Design review of the part built by this model. Coordinates are the model's own, in mm. Face numbers are marked on the shaded views. A direction names the side the tool comes from. Coordinates: 2 decimals unless noted, no trailing zeros. Write each loop counter-clockwise with the first axis right and the second up, starting at its lowest first coordinate (ties: lowest second). Pieces come first, ordered by that corner, then holes. Notation, with made-up numbers: (37, 63) -> (46, 63) arc R27 cw to (46, 80) -> close; hole circle Ø5 at (-29.75, 11.25). An arc over 180 degrees is marked (long way). Answer in a Markdown table with one row per item. Add a question column.
Item 1: Clearance check with flat-ended pins moving along their axes: P1, Ø4, axis at x = 12.7, z = -12.7, coming from the -Y side; P2, Ø2, axis at x = 5.5, z = -1, coming from the +Y side; P3, Ø1.5, axis at x = 15.5, y = -16, coming from the -Z side; P4, Ø5.5, axis at x = 8, z = -10, coming from the +Y side. State where each tip first meets the part, or that it passes through.
Item 2: Draft analysis for pull direction X (two halves, no side actions). For the marked faces 1, 2, 3 and 4, state which applies: released by +X, released by -X, zero draft, split by the parting line, or undercut.
Item 3: Take a section at A-A, the plane z = -12.7. Write out the cut boundary in (x, y).
Item 4: Take a section at C-C, the plane x = 12.7. Write out the cut boundary in (y, z).
Item 5: Take a section at D-D, the plane y = -22. Write out the cut boundary in (x, z), and give its area (3 significant figures).
Item 6: To check wall thickness, follow line 1 (Y direction, x = 12.7, z = -0.5); line 2 (X direction, y = -22, z = -12.7); line 3 (Z direction, x = 16.75, y = -1.5). State the ranges of each line that lie inside material, in increasing order.
Item 7: Take a section at B-B, the plane y = -12.7. Write out the cut boundary in (x, z), and give its area (3 significant figures).
Item 8: For the marked faces 5 and 6, list the 3-axis set-ups (+Z, -Z, +X, -X, +Y, -Y) from which the entire face can be reached by the end or side of a thin tool; tool diameter is ignored.
from build123d import *

# Parameters (mm, degrees)
SKETCH1_W           = 25.4
SKETCH1_H           = 25.4
SKETCH1_R           = 3.429
BOSS_EXTRUDE1_DEPTH = 2.54
SKETCH3_W           = 25.4
SKETCH3_H           = 5.08
BOSS_EXTRUDE2_DEPTH = 25.4
SKETCH4_R           = 3.429
CUT_EXTRUDE1_DEPTH  = 5.08
FILLET1_R           = 2.54


with BuildPart() as part:
    # Sketch1 → Boss-Extrude1 (new, symmetric)
    with BuildSketch(Plane.XY):
        with Locations((12.7, -12.7)):
            Rectangle(SKETCH1_W, SKETCH1_H)
        with Locations((12.7, -12.7)):
            Circle(SKETCH1_R, mode=Mode.SUBTRACT)
    extrude(amount=BOSS_EXTRUDE1_DEPTH, both=True)

    # Sketch3 → Boss-Extrude2 (add)
    with BuildSketch(Plane.XY.offset(2.54)):
        with Locations((12.7, -22.86)):
            Rectangle(SKETCH3_W, SKETCH3_H)
    extrude(amount=-BOSS_EXTRUDE2_DEPTH)

    # Sketch4 → Cut-Extrude1 (cut)
    with BuildSketch(Plane(origin=(0, -20.32, 0), x_dir=(1, 0, 0), z_dir=(0, 1, 0))):
        with Locations(Location((12.7, 12.7, 0), (0, 0, 270))):
            Circle(SKETCH4_R)
    extrude(amount=-CUT_EXTRUDE1_DEPTH, mode=Mode.SUBTRACT)

    # Fillet1
    fillet1_edges = [part.edges().sort_by_distance(p)[0] for p in [
        (12.7, -20.32, -2.54),
    ]]
    fillet(fillet1_edges, radius=FILLET1_R)


solid = part.part
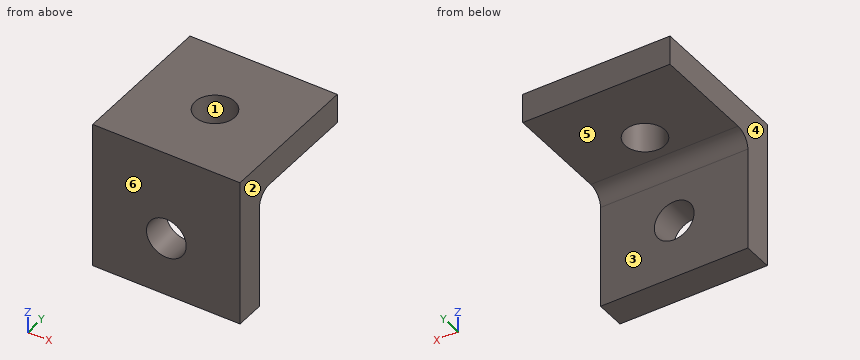
Answers:
| question | item | result |
|---|---|---|
| 1 | P1 | passes through |
| 1 | P2 | stops at y = 0 |
| 1 | P3 | stops at z = -2.54 |
| 1 | P4 | stops at y = -20.32 |
| 2 | face 1 | undercut |
| 2 | face 2 | released by +X |
| 2 | face 3 | zero draft |
| 2 | face 4 | released by -X |
| 3 | outline | (0, -25.4) -> (9.27, -25.4) -> (9.27, -20.32) -> (0, -20.32) -> close; (16.13, -25.4) -> (25.4, -25.4) -> (25.4, -20.32) -> (16.13, -20.32) -> close |
| 4 | outline | (-25.4, -22.86) -> (-20.32, -22.86) -> (-20.32, -16.13) -> (-25.4, -16.13) -> close; (-25.4, -9.27) -> (-20.32, -9.27) -> (-20.32, -5.08) arc R2.54 cw to (-17.78, -2.54) -> (-16.13, -2.54) -> (-16.13, 2.54) -> (-25.4, 2.54) -> close; (-9.27, -2.54) -> (0, -2.54) -> (0, 2.54) -> (-9.27, 2.54) -> close |
| 5 | outline | (0, -22.86) -> (25.4, -22.86) -> (25.4, 2.54) -> (0, 2.54) -> close; hole circle Ø6.86 at (12.7, -12.7) |
| 5 | area | 608 mm^2 |
| 6 | line 1 | y = -25.4 to -16.13, -9.27 to 0 |
| 6 | line 2 | x = 0 to 9.27, 16.13 to 25.4 |
| 6 | line 3 | z = -2.54 to 2.54 |
| 7 | outline | (0, -2.54) -> (9.27, -2.54) -> (9.27, 2.54) -> (0, 2.54) -> close; (16.13, -2.54) -> (25.4, -2.54) -> (25.4, 2.54) -> (16.13, 2.54) -> close |
| 7 | area | 94.2 mm^2 |
| 8 | face 5 | -Z, +X, -X, +Y |
| 8 | face 6 | +Z, -Z, +X, -X, -Y |
